Read the model definition and answer for the solid it produces. Units are mm, in the model's axes. A direction names the side the tool comes from. Coordinates: 2 decimals unless noted, no trailing zeros. Loops run counter-clockwise (first coordinate to the right, second up) from the corner with the lowest first, then second, coordinate; pieces in that order, holes last.
Q1. The mould has two halves that part along X. Classify faces 4 (the face through (3, 45, 9)), 5 (the face through (2.703, 22.815, 8.584)), 6 (the face through (14.18, 2.46, -1.86)): pulls with the +X half, pulls with the -X half, needs draft (parallel to the pull), parting line crosses it, or undercut.
Q2. Section C-C (x = 0) is taken. Give the vertices of the cut face in (y, z), then the cut area to 3 significant figures.
Q3. Section D-D (z = 7.75) is taken. Give the vertices of the cut face in (x, y).
Q4. Straight lines are drawn through the part: line 1 (X direction, y = 30, z = 0); line 2 (Z direction, x = 0, y = 13); line 3 (Y direction, x = -11.75, z = 3.5). For each, find the intervals that lie inside material, in ascending order.
Q5. Flat-ended cylindrical pins translate along their axes: P1, Ø6, axis at y = 21.5, z = -6.5, coming from the -X side; P2, Ø4, axis at y = 21, z = -10.5, coming from the +X side; P3, Ø1, axis at x = 4, y = 22.5, coming from the -Z side. Find the tip coordinate at first contact, or state that the pin passes through.
Q6. Section B-B (x = -4.75) is taken. Give the vertices of the cut face in (y, z).
Q7. Section A-A (z = 0) is taken. Give the vertices of the cut face in (x, y), then the cut area to 3 significant figures.
Q8. Which of the six approach directions +Z, -Z, +X, -X, +Y, -Y give full straight-line access (tool end or side, diameter ignored) to faces 1 (the face through (0, 25, 12)), 2 (the face through (-9.3, 0, 0.2)), 3 (the face through (7.5, 25.3, -7.3))?
from build123d import *

# Parameters (mm, degrees)
SKETCH1_R           = 14.3
BOSS_EXTRUDE1_DEPTH = 5
SKETCH2_R           = 12
BOSS_EXTRUDE2_DEPTH = 45
SKETCH3_R           = 9
CUT_EXTRUDE1_DEPTH  = 50.33538284
CUT_EXTRUDE3_DEPTH  = 40


with BuildPart() as part:
    # Sketch1 → Boss-Extrude1 (new body)
    with BuildSketch(Plane(origin=(0, 0, 0), x_dir=(1, 0, 0), z_dir=(0, 1, 0))):
        with Locations(Location((0, 0, 0), (0, 0, 270))):
            Circle(SKETCH1_R)
    extrude(amount=BOSS_EXTRUDE1_DEPTH)

    # Sketch2 → Boss-Extrude2 (add)
    with BuildSketch(Plane.XZ):
        with Locations(Location((0, 0, 0), (0, 0, 270))):
            Circle(SKETCH2_R)
    extrude(amount=-BOSS_EXTRUDE2_DEPTH)

    # Sketch3 → Cut-Extrude1 (cut, through all)
    with BuildSketch(Plane(origin=(0, 45, 0), x_dir=(1, 0, 0), z_dir=(0, 1, 0))):
        with Locations(Location((0, 0, 0), (0, 0, 270))):
            Circle(SKETCH3_R)
    extrude(amount=-CUT_EXTRUDE1_DEPTH, mode=Mode.SUBTRACT)

    # Sketch4 → Cut-Extrude3 (cut)
    with BuildSketch(Plane(origin=(0, 45, 0), x_dir=(1, 0, 0), z_dir=(0, 1, 0))):
        with BuildLine():
            Line((-8.842350879, 9.578144326), (-2.340207376, 2.534941703))
            ThreePointArc((-2.340207376, 2.534941703), (0, 3.45), (2.340207376, 2.534941703))
            Line((2.340207376, 2.534941703), (9.389352033, 9.042570774))
            ThreePointArc((9.389352033, 9.042570774), (0.382769282, 13.030023234), (-8.842350879, 9.578144326))
        make_face()
    extrude(amount=-CUT_EXTRUDE3_DEPTH, mode=Mode.SUBTRACT)


solid = part.part
Numbers:
1. face 4: needs draft
1. face 5: undercut
1. face 6: parting line crosses it
2. outline: (0, -14.3) - (5, -14.3) - (5, -9) - (0, -9) - close; (0, 9) - (45, 9) - (45, 12) - (5, 12) - (5, 14.3) - (0, 14.3) - close
2. area: 173 mm2
3. outline: (-12.02, 0) - (-4.58, 0) - (-4.58, 45) - (-9.16, 45) - (-9.16, 5) - (-12.02, 5) - close; (4.58, 0) - (12.02, 0) - (12.02, 5) - (9.16, 5) - (9.16, 45) - (4.58, 45) - close
4. line 1: x = -12 to -9, 9 to 12
4. line 2: z = 9 to 12
4. line 3: y = 0 to 5
5. P1: stops at x = -11.48
5. P2: stops at x = -7.85
5. P3: stops at z = 7.79
6. outline: (0, -13.49) - (5, -13.49) - (5, -7.64) - (0, -7.64) - close; (0, 7.64) - (45, 7.64) - (45, 11.02) - (5, 11.02) - (5, 13.49) - (0, 13.49) - close
7. outline: (-14.3, 0) - (-9, 0) - (-9, 45) - (-12, 45) - (-12, 5) - (-14.3, 5) - close; (9, 0) - (14.3, 0) - (14.3, 5) - (12, 5) - (12, 45) - (9, 45) - close
7. area: 293 mm2
8. face 1: +Y
8. face 2: +Z, -Z, +X, -X, -Y
8. face 3: -Z, +Y
